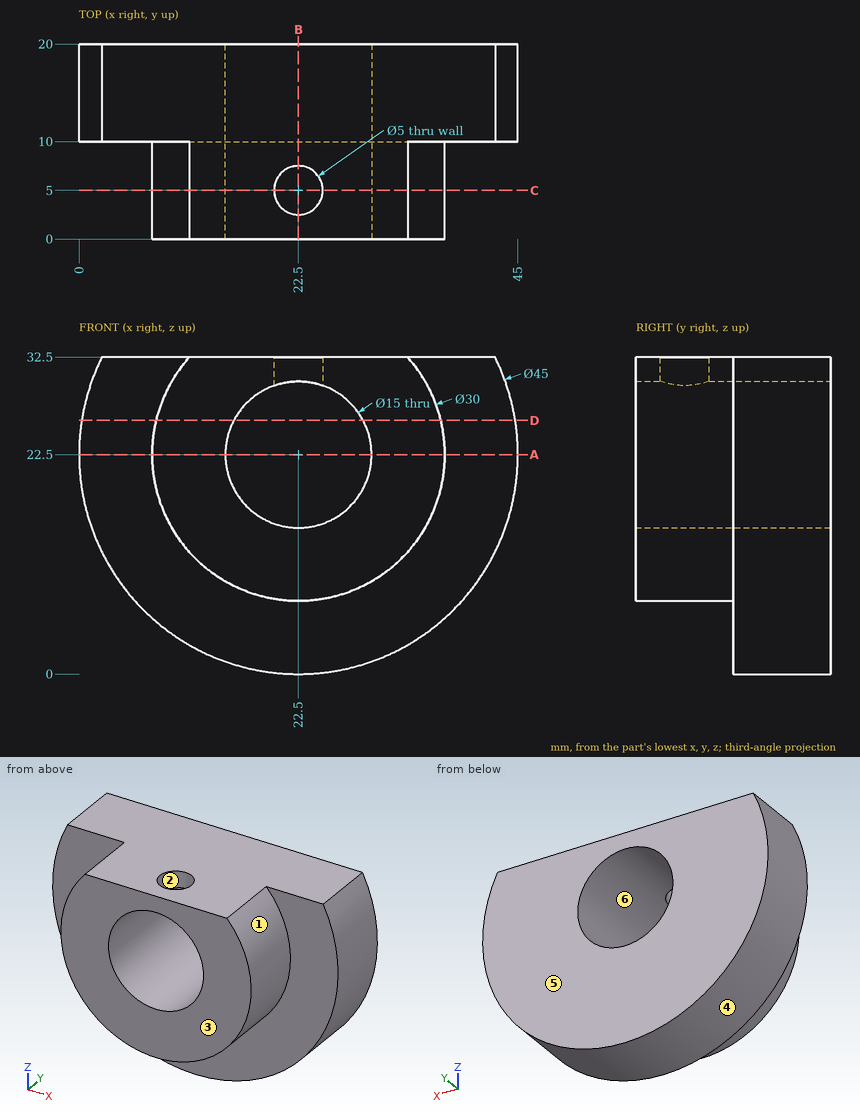
Check sheet for the drawn part. Datum: minimum x, y, z corner. Units: mm. A direction names the side the tool comes from. Round coordinates to 2 decimals unless told otherwise and drop trailing zeros. Write each loop counter-clockwise with the first axis right and the second up, starting at its lowest first coordinate (ties: lowest second). Pieces come first, ordered by that corner, then holes. Notation, with made-up numbers: (-26, -8) -> (13, -8) arc R19 cw to (13, 25) -> close; hole circle Ø10 at (35.5, 39). An arc over 180 degrees is marked (long way). Write each question's results on one line, items separated by ' | '.
Q1. Draft check along X on the marked faces 4, 5 and 6. Enter one of: released by +X, released by -X, zero draft, split by the parting line, or undercut.
Derived:
face 4: split by the parting line | face 5: zero draft | face 6: undercut
Q2. Sectioned sample at A-A, the plane z = 22.5. Record the boundary of the cut face in (x, y), and give its area (3 significant figures).
Derived:
outline: (0, 10) -> (7.5, 10) -> (7.5, 0) -> (15, 0) -> (15, 20) -> (0, 20) -> close; (30, 0) -> (37.5, 0) -> (37.5, 10) -> (45, 10) -> (45, 20) -> (30, 20) -> close | area: 450 mm²
Q3. Access from +Z, -Z, +X, -X, +Y, -Y to the whole of each face (thin tool, end or side, straight path). Record for the marked faces 1, 2 and 3.
Derived:
face 1: -Y | face 2: +Z | face 3: +Z, -Z, +X, -X, -Y
Q4. Sectioned sample at C-C, the plane y = 5. Record the boundary of the cut face in (x, z), and give its area (4 significant figures).
Derived:
outline: (11.32, 32.5) arc R15 ccw (long way) to (33.68, 32.5) -> (25, 32.5) -> (25, 29.57) arc R7.5 cw (long way) to (20, 29.57) -> (20, 32.5) -> close | area: 439.5 mm²
Q5. Sectioned sample at B-B, the plane x = 22.5. Record the boundary of the cut face in (y, z), and give its area (4 significant figures).
Derived:
outline: (0, 7.5) -> (10, 7.5) -> (10, 0) -> (20, 0) -> (20, 15) -> (0, 15) -> close; (0, 30) -> (2.5, 30) -> (2.5, 32.5) -> (0, 32.5) -> close; (7.5, 30) -> (20, 30) -> (20, 32.5) -> (7.5, 32.5) -> close | area: 262.5 mm²
Q6. Thickness scan on probe 1 along Y at (x, z) = (22.5, 30.2); probe 2 along Z at (x, y) = (22.5, 6.25); probe 3 along Y at (x, z) = (22, 31). Record the ranges inside material, lowest first.
Derived:
probe 1: y = 0 to 2.5, 7.5 to 20 | probe 2: z = 7.5 to 15 | probe 3: y = 0 to 2.55, 7.45 to 20
Q7. Go/stop test with flat-tipped pins: pin 1 Ø1 at (y, z) = (4.5, 15.5) entering from +X; pin 2 Ø1 at (y, z) = (15.5, 17.5) entering from +X; pin 3 Ø10 at (x, z) = (22.5, 22.5) entering from -Y; pin 4 Ø1.5 at (y, z) = (17.5, 26.5) entering from -X. Record where each tip stops, or that it passes through.
Derived:
pin 1: stops at x = 36.02 | pin 2: stops at x = 44.55 | pin 3: passes through | pin 4: stops at x = 0.24
Q8. Sectioned sample at D-D, the plane z = 26. Record the boundary of the cut face in (x, y).
Derived:
outline: (0.27, 10) -> (7.91, 10) -> (7.91, 0) -> (15.87, 0) -> (15.87, 20) -> (0.27, 20) -> close; (29.13, 0) -> (37.09, 0) -> (37.09, 10) -> (44.73, 10) -> (44.73, 20) -> (29.13, 20) -> close
